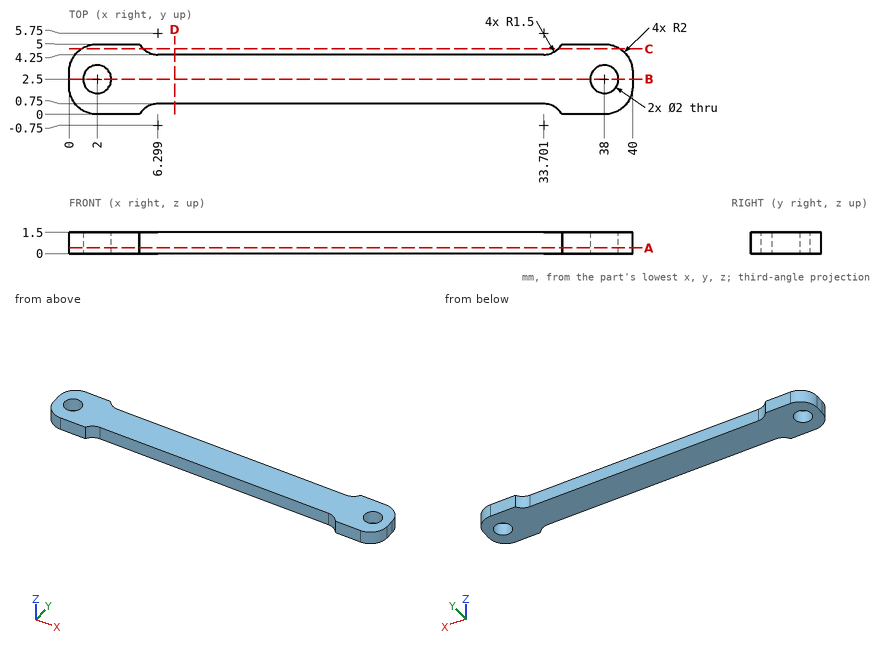
Part print with two shaded views. Sizes in mm from the minimum x, y, z corner. Give positions to 0.01 mm unless a question says otherwise; leave off trailing zeros. Order: outer loops, then holes, each group sorted by start corner. A loop starts at its lowest first (then second) coordinate and runs counter-clockwise, first axis right, second up. Notation, with made-up numbers: M 23.25,64.5 L 81.25,64.5 A18 cw 81.25,70.5 Z; hole C -4.5,37 d7. An arc over 180 degrees is marked long. Put each result on its own line as item: value.
Item 1: Cut at A-A on z = 0.4. Write the cut outline in (x, y).
Results are:
outline: M 0,2 A2 ccw 2,0 L 5,0 A1.5 cw 6.3,0.75 L 33.7,0.75 A1.5 cw 35,0 L 38,0 A2 ccw 40,2 L 40,3 A2 ccw 38,5 L 35,5 A1.5 cw 33.7,4.25 L 6.3,4.25 A1.5 cw 5,5 L 2,5 A2 ccw 0,3 Z; hole C 2,2.5 d2; hole C 38,2.5 d2
Item 2: Cut at B-B on y = 2.5. Write the cut outline in (x, z), then the cut area to 3 significant figures.
Results are:
outline: M 0,0 L 1,0 L 1,1.5 L 0,1.5 Z; M 3,0 L 37,0 L 37,1.5 L 3,1.5 Z; M 39,0 L 40,0 L 40,1.5 L 39,1.5 Z
area: 54.0 mm2
Item 3: Cut at C-C on y = 4.65. Write the cut outline in (x, z).
Results are:
outline: M 0.87,0 L 5.28,0 L 5.28,1.5 L 0.87,1.5 Z; M 34.72,0 L 39.13,0 L 39.13,1.5 L 34.72,1.5 Z
Item 4: Wall check: probe 1 along Y at (x, z) = (38, 1.15); probe 2 along X at (y, z) = (3.3, 0.65); probe 3 along Y at (x, z) = (11.5, 0.5). Give the ranges that are in metal, low to high.
Results are:
probe 1: 0 to 1.5, 3.5 to 5
probe 2: 0.02 to 1.4, 2.6 to 37.4, 38.6 to 39.98
probe 3: 0.75 to 4.25
Item 5: Cut at D-D on x = 7.5. Write the cut outline in (y, z).
Results are:
outline: M 0.75,0 L 4.25,0 L 4.25,1.5 L 0.75,1.5 Z
Item 6: Drop flat-ended pins along their axis: pin 1 Ø0.8 at (x, z) = (24.5, 1) entering from +Y; pin 2 Ø1.6 at (x, y) = (2, 2.5) entering from +Z. Give the stop position or say it passes through.
Results are:
pin 1: y = 4.25
pin 2: through
